```python
from build123d import *

# Parameters (mm, degrees)
SKETCH1_R                = 45
SKETCH1_R_2              = 42.5
BOSS_EXTRUDE1_DEPTH      = 120
SKETCH2_R                = 2.5
BOSS_EXTRUDE2_DEPTH      = 5
FILLET2_R                = 3
CIRPATTERN1_COUNT        = 4
FILLET2_OF_CIRPATTERN1_R = 3
MIRROR1_START            = 115
MIRROR1_OUTLINE_R        = 2.5
MIRROR1_DEPTH            = 5
SKETCH1_2_R              = 42.5
BOSS_EXTRUDE4_DEPTH      = 15
SKETCH7_R                = 2
CUT_EXTRUDE1_DEPTH       = 144.003496461
SKETCH10_R               = 20
CUT_EXTRUDE5_DEPTH       = 10
BOSS_EXTRUDE3_DEPTH      = 120
CIRPATTERN2_COUNT        = 4
FILLET1_R                = 10


# Read off the part's stored shape, not the designer's step: Mirror1
with BuildPart() as part:
    # Sketch1 → Boss-Extrude1 (new body)
    with BuildSketch(Plane(origin=(0, 0, 0), x_dir=(1, 0, 0), z_dir=(0, 1, 0))):
        with Locations(Location((0, 0, 0), (0, 0, 270))):
            Circle(SKETCH1_R)
        with Locations(Location((0, 0, 0), (0, 0, 270))):
            Circle(SKETCH1_R_2, mode=Mode.SUBTRACT)
    extrude(amount=BOSS_EXTRUDE1_DEPTH)

    # Sketch2 → Boss-Extrude2 (add)
    with BuildSketch(Plane(origin=(0, 0, 0), x_dir=(1, 0, 0), z_dir=(0, 1, 0))):
        with BuildLine():
            Line((-5, -44.72135955), (-5, -50))
            ThreePointArc((-5, -50), (0, -55), (5, -50))
            Line((5, -50), (5, -44.72135955))
            ThreePointArc((5, -44.72135955), (0, -45), (-5, -44.72135955))
        make_face()
        with Locations(Location((0, -50, 0), (0, 0, 270))):
            Circle(SKETCH2_R, mode=Mode.SUBTRACT)
    boss_extrude2 = extrude(amount=BOSS_EXTRUDE2_DEPTH)

    # Fillet2
    fillet2_edges = [part.edges().sort_by_distance(p)[0] for p in [
        (5, 2.5, 44.72135955),
        (-5, 2.5, 44.72135955),
    ]]
    fillet(fillet2_edges, radius=FILLET2_R)

    # CirPattern1: Boss-Extrude2 ×4 about axis
    cirpattern1_axis = Axis((0, 0, 0), (0, 1, 0))
    for i in range(1, CIRPATTERN1_COUNT):
        add(boss_extrude2.rotate(cirpattern1_axis, i * 360 / CIRPATTERN1_COUNT))

    # Fillet2 of CirPattern1
    fillet2_of_cirpattern1_edges = [part.edges().sort_by_distance(p)[0] for p in [
        (44.72135955, 2.5, -5),
        (44.72135955, 2.5, 5),
        (-5, 2.5, -44.72135955),
        (5, 2.5, -44.72135955),
        (-44.72135955, 2.5, 5),
        (-44.72135955, 2.5, -5),
    ]]
    fillet(fillet2_of_cirpattern1_edges, radius=FILLET2_OF_CIRPATTERN1_R)

    # Mirror1 outline → Mirror1 (add)
    # profile 1 of 4: a face of its own
    with BuildSketch(Plane(origin=(0, 0, 0), x_dir=(1, 0, 0), z_dir=(0, 1, 0)).offset(MIRROR1_START)):
        with BuildLine():
            ThreePointArc((-7.5, -44.370598373), (-5.708712153, -45.392146592), (-5, -47.328638265))
            Line((-5, -47.328638265), (-5, -50))
            ThreePointArc((-5, -50), (0, -55), (5, -50))
            Line((5, -50), (5, -47.328638265))
            ThreePointArc((5, -47.328638265), (5.708712153, -45.392146592), (7.5, -44.370598373))
            ThreePointArc((7.5, -44.370598373), (0, -45), (-7.5, -44.370598373))
        make_face()
        with Locations((0, -50)):
            Circle(MIRROR1_OUTLINE_R, mode=Mode.SUBTRACT)
    # profile 2 of 4: a face of its own
    with BuildSketch(Plane(origin=(0, 0, 0), x_dir=(1, 0, 0), z_dir=(0, 1, 0)).offset(MIRROR1_START)):
        with BuildLine():
            ThreePointArc((-47.328638265, -5), (-45.392146592, -5.708712153), (-44.370598373, -7.5))
            ThreePointArc((-44.370598373, -7.5), (-45, 0), (-44.370598373, 7.5))
            ThreePointArc((-44.370598373, 7.5), (-45.392146592, 5.708712153), (-47.328638265, 5))
            Line((-47.328638265, 5), (-50, 5))
            ThreePointArc((-50, 5), (-55, 0), (-50, -5))
            Line((-50, -5), (-47.328638265, -5))
        make_face()
        with Locations((-50, 0)):
            Circle(MIRROR1_OUTLINE_R, mode=Mode.SUBTRACT)
    # profile 3 of 4: a face of its own
    with BuildSketch(Plane(origin=(0, 0, 0), x_dir=(1, 0, 0), z_dir=(0, 1, 0)).offset(MIRROR1_START)):
        with BuildLine():
            ThreePointArc((44.370598373, 7.5), (45, 0), (44.370598373, -7.5))
            ThreePointArc((44.370598373, -7.5), (45.392146592, -5.708712153), (47.328638265, -5))
            Line((47.328638265, -5), (50, -5))
            ThreePointArc((50, -5), (55, 0), (50, 5))
            Line((50, 5), (47.328638265, 5))
            ThreePointArc((47.328638265, 5), (45.392146592, 5.708712153), (44.370598373, 7.5))
        make_face()
        with Locations((50, 0)):
            Circle(MIRROR1_OUTLINE_R, mode=Mode.SUBTRACT)
    # profile 4 of 4: a face of its own
    with BuildSketch(Plane(origin=(0, 0, 0), x_dir=(1, 0, 0), z_dir=(0, 1, 0)).offset(MIRROR1_START)):
        with BuildLine():
            ThreePointArc((-5, 47.328638265), (-5.708712153, 45.392146592), (-7.5, 44.370598373))
            ThreePointArc((-7.5, 44.370598373), (0, 45), (7.5, 44.370598373))
            ThreePointArc((7.5, 44.370598373), (5.708712153, 45.392146592), (5, 47.328638265))
            Line((5, 47.328638265), (5, 50))
            ThreePointArc((5, 50), (0, 55), (-5, 50))
            Line((-5, 50), (-5, 47.328638265))
        make_face()
        with Locations((0, 50)):
            Circle(MIRROR1_OUTLINE_R, mode=Mode.SUBTRACT)
    extrude(amount=MIRROR1_DEPTH)

    # Sketch1<2> → Boss-Extrude4 (add)
    with BuildSketch(Plane(origin=(0, 0, 0), x_dir=(1, 0, 0), z_dir=(0, 1, 0))):
        with Locations(Location((0, 0, 0), (0, 0, 270))):
            Circle(SKETCH1_2_R)
    extrude(amount=BOSS_EXTRUDE4_DEPTH)

    # Sketch7 → Cut-Extrude1 (cut, through all)
    with BuildSketch(Plane.XZ):
        with Locations(Location((0, 0, 0), (0, 0, 270))):
            Circle(SKETCH7_R)
    extrude(amount=-CUT_EXTRUDE1_DEPTH, mode=Mode.SUBTRACT)

    # Sketch10 → Cut-Extrude5 (cut)
    with BuildSketch(Plane.XZ):
        with Locations(Location((0, 0, 0), (0, 0, 270))):
            Circle(SKETCH10_R)
    extrude(amount=-CUT_EXTRUDE5_DEPTH, mode=Mode.SUBTRACT)

    # Sketch6 → Boss-Extrude3 (add)
    with BuildSketch(Plane.XZ):
        with BuildLine():
            Line((-22.588713996, -36), (22.588713996, -36))
            ThreePointArc((22.588713996, -36), (0, -42.5), (-22.588713996, -36))
        make_face()
    boss_extrude3 = extrude(amount=-BOSS_EXTRUDE3_DEPTH)

    # CirPattern2: Boss-Extrude3 ×4 about axis
    cirpattern2_axis = Axis((0, 0, 0), (0, 1, 0))
    for i in range(1, CIRPATTERN2_COUNT):
        add(boss_extrude3.rotate(cirpattern2_axis, i * 360 / CIRPATTERN2_COUNT))

    # Fillet1
    fillet1_edges = [part.edges().sort_by_distance(p)[0] for p in [
        (-22.588713996, 67.5, -36),
        (22.588713996, 67.5, -36),
        (-36, 67.5, 22.588713996),
        (-36, 67.5, -22.588713996),
        (22.588713996, 67.5, 36),
        (-22.588713996, 67.5, 36),
        (36, 67.5, -22.588713996),
        (36, 67.5, 22.588713996),
    ]]
    fillet(fillet1_edges, radius=FILLET1_R)


solid = part.part
```
The model under review builds one solid part; all positions refer to its coordinate system, in mm. A direction names the side the tool comes from. Coordinates: 2 decimals unless noted, no trailing zeros. Order: outer loops, then holes, each group sorted by start corner. A loop starts at its lowest first (then second) coordinate and runs counter-clockwise, first axis right, second up. Notation, with made-up numbers: (88, -28.75) -> (114, -28.75) arc R25 cw to (114, 8.25) -> close; hole circle Ø3 at (84.5, 83.5). An arc over 180 degrees is marked (long way). Answer in a Markdown table with one row per item. Add a question column.
Item 1: We need section B-B on x = 0. Give the number of separate pieces and of enclosed holes in the cut face, plus the area to 3 significant figures.
Item 2: We need section D-D on x = -38. Write out the cut boundary in (y, z).
Item 3: We need section A-A on y = 72. Write out the cut boundary in (x, z), plus the area to 3 significant figures.
Item 4: Mouldability with a two-part tool opening along X and no side actions: class faces 3 (the flat face through (36, 67, 0)), 4 (the cylindrical face through (5.7, 2.5, 45.4)), 5 (the flat face through (-0.3, 120, 36.4)), 6 (the cylindrical face through (35.472, 68.235, 22.705)) as +X half, -X half, draft (parallel to the pull), parting line (faces both ways), or undercut.
Item 5: Machinability: for faces 1 (the cylindrical face through (-55, 117, 0)), 2 (the cylindrical face through (-22.705, 68.235, -35.472)), which of the approach directions +Z, -Z, +X, -X, +Y, -Y give a long, thin tool a straight path to every point of the face, cutting with its end or side? Answer none if there is none.
Item 6: Clearance check with flat-ended pins moving along their axes: pin 1 (8 mm diameter, centred on y = 71.5, z = -26, fed in from -X); pin 2 (8 mm diameter, centred on x = 6, z = 15.5, fed in from -Y); pin 3 (1.5 mm diameter, centred on y = 67.5, z = 9, fed in from -X); pin 4 (3 mm diameter, centred on y = 117.5, z = -48.5, fed in from -X). State where each tip first meets the part, or that it passes through.
Item 7: We need section C-C on z = -10. Write out the cut boundary in (x, y), plus the area to 3 significant figures.
Item 8: To check wall thickness, follow probe 1 along Z at (x, y) = (0, 117); probe 2 along X at (y, z) = (3.85, 50). State the ranges of each line that lie inside material, in increasing order.
Final values:
| question | item | result |
|---|---|---|
| 1 | separate pieces | 6 |
| 1 | enclosed holes | 0 |
| 1 | area | 2,920 mm2 |
| 2 | outline | (0, -24.1) -> (120, -24.1) -> (120, 24.1) -> (0, 24.1) -> close |
| 3 | outline | circle Ø90 at (0, 0); hole (-36, -19.5) arc R10 ccw to (-34, -25.5) arc R42.5 ccw to (-25.5, -34) arc R10 ccw to (-19.5, -36) -> (19.5, -36) arc R10 ccw to (25.5, -34) arc R42.5 ccw to (34, -25.5) arc R10 ccw to (36, -19.5) -> (36, 19.5) arc R10 ccw to (34, 25.5) arc R42.5 ccw to (25.5, 34) arc R10 ccw to (19.5, 36) -> (-19.5, 36) arc R10 ccw to (-25.5, 34) arc R42.5 ccw to (-34, 25.5) arc R10 ccw to (-36, 19.5) -> close |
| 3 | area | 1,490 mm2 |
| 4 | face 3 | undercut |
| 4 | face 4 | +X half |
| 4 | face 5 | draft |
| 4 | face 6 | undercut |
| 5 | face 1 | -X, +Y, -Y |
| 5 | face 2 | +Y |
| 6 | pin 1 | stops at x = -39.26 |
| 6 | pin 2 | stops at y = 0 |
| 6 | pin 3 | stops at x = -44.24 |
| 6 | pin 4 | stops at x = -5.02 |
| 7 | outline | (-43.87, 0) -> (-17.32, 0) -> (-17.32, 10) -> (17.32, 10) -> (17.32, 0) -> (43.87, 0) -> (43.87, 120) -> (36, 120) -> (36, 15) -> (-36, 15) -> (-36, 120) -> (-43.87, 120) -> close |
| 7 | area | 2,620 mm2 |
| 8 | probe 1 | z = -55 to -52.5, -47.5 to -36, 36 to 47.5, 52.5 to 55 |
| 8 | probe 2 | x = -5 to -2.5, 2.5 to 5 |
